Can you work these out from the model? Positions are in its coordinate system, mm. A direction names the side the tool comes from. Give positions to 0.01 mm unless a question says otherwise; leave off trailing zeros. Loops run counter-clockwise (first coordinate to the right, second up) from the corner with the lowest first, then second, coordinate; pieces in that order, holes last. Notation, with made-up numbers: (83, -33.5) - (104, -33.5) arc R32 cw to (104, -4.5) - close; hole circle Ø11 at (4, -9.5). An arc over 180 degrees is marked (long way). Write item = value, one per line.
Autodesk Inventor part; units mm, degrees
ref_plane "YZ Plane" through (0, 0, 0) normal (1, 0, 0) x (0, 1, 0)
ref_plane "XZ Plane" through (0, 0, 0) normal (0, 1, 0) x (-1, 0, 0)
ref_plane "XY Plane" through (0, 0, 0) normal (0, 0, 1) x (1, 0, 0)
sketch "Sketch1" plane through (0, 0, 0) normal (1, 0, 0) x (0, 1, 0)
  line L0 (-1.5, 6.858) -> (1.5, 6.858)
  line L1 (1.5, 6.858) -> (1.5, -6.858)
  line L2 (1.5, -6.858) -> (-1.5, -6.858)
  line L3 (-1.5, -6.858) -> (-1.5, 6.858)
  line L4 (-1.5, 6.858) -> (1.5, -6.858) construction
  line L5 (1.5, 6.858) -> (-1.5, -6.858) construction
  line L6 (1.5, 6.858) -> (39.5, 6.858)
  line L7 (39.5, 6.858) -> (39.5, 9.858)
  line L8 (39.5, 9.858) -> (1.5, 9.858)
  line L9 (1.5, 9.858) -> (1.5, 6.858)
  line L10 (1.5, -6.858) -> (39.5, -6.858)
  line L11 (39.5, -6.858) -> (39.5, -9.858)
  line L12 (39.5, -9.858) -> (1.5, -9.858)
  line L13 (1.5, -9.858) -> (1.5, -6.858)
  line L14 (9.5, 6.858) -> (1.5, 6.858)
  line L15 (1.5, 6.858) -> (1.5, -0.142)
  line L16 (1.5, -0.142) -> (9.5, -0.142)
  line L17 (9.5, -0.142) -> (9.5, 6.858)
  line L18 (9.5, -6.858) -> (1.5, -6.858)
  line L19 (1.5, -6.858) -> (1.5, -0.142)
  line L20 (1.5, -0.142) -> (9.5, -0.142)
  line L21 (9.5, -0.142) -> (9.5, -6.858)
  line L22 (9.5, -0.142) -> (1.5, -0.142)
  line L23 (1.5, 6.858) -> (-1.5, 6.858)
  line L24 (-1.5, 6.858) -> (-1.5, 9.858)
  line L25 (-1.5, 9.858) -> (1.5, 9.858)
  line L26 (1.5, 9.858) -> (1.5, 6.858)
  line L27 (1.5, -6.858) -> (-1.5, -6.858)
  line L28 (-1.5, -6.858) -> (-1.5, -9.858)
  line L29 (-1.5, -9.858) -> (1.5, -9.858)
  line L30 (1.5, -9.858) -> (1.5, -6.858)
  point P0 (0, 0)
  dimension "d0" = 3
  dimension "d2" = 13.716
  dimension "d3" = 3
  dimension "d4" = 3
  dimension "d5" = 38
  dimension "d6" = 38
  dimension "d7" = 0
  dimension "d8" = 8
  dimension "d9" = 8
  dimension "d12" = 7
  dimension "d13" = 6.716
extrude "Extrusion1" add sketch "Sketch1" along normal blind 45
sketch "Sketch2" plane through (0, -1.5, 9.858) normal (0, 0, 1) x (1, 0, 0)
  line L0 (5, 7) -> (8.9446, 7)
  arc A0 (5, 7) -> (5, 0) centre (5, 3.5) ccw
  line L1 (8.9446, 0) -> (5, 0)
  arc A1 (13.3822, 14.1239) -> (31.6178, 14.1239) centre (22.5, 3.5) ccw
  line L2 (13.3822, 14.1239) -> (13.3822, 15.7096)
  line L3 (13.6751, 16.4167) -> (15.15, 17.8916)
  arc A2 (13.6751, 16.4167) -> (13.3822, 15.7096) centre (14.3822, 15.7096) ccw
  arc A3 (16.15, 20.3916) -> (15.15, 19.3916) centre (16.15, 19.3916) ccw
  line L4 (15.15, 19.3916) -> (15.15, 17.8916)
  line L5 (28.85, 20.3916) -> (16.15, 20.3916)
  arc A4 (29.85, 19.3916) -> (28.85, 20.3916) centre (28.85, 19.3916) ccw
  line L6 (29.85, 17.8916) -> (29.85, 19.3916)
  line L7 (31.3249, 16.4167) -> (29.85, 17.8916)
  line L8 (31.6178, 15.7096) -> (31.6178, 14.1239)
  arc A5 (31.6178, 15.7096) -> (31.3249, 16.4167) centre (30.6178, 15.7096) ccw
  line L9 (40, 7) -> (36.0554, 7)
  arc A6 (40, 0) -> (40, 7) centre (40, 3.5) ccw
  line L10 (36.0554, 0) -> (40, 0)
  line L11 (40, 7) -> (36.0554, 7)
  arc A7 (40, 0) -> (40, 7) centre (40, 3.5) ccw
  line L12 (36.0554, 0) -> (40, 0)
  line L13 (8.9446, 0) -> (5, 0)
  line L14 (36.0554, 0) -> (40, 0)
  line L15 (0, 41) -> (0, 0)
  line L16 (0, 0) -> (45, 0)
  line L17 (45, 41) -> (45, 0)
  line L18 (0, 41) -> (45, 41)
  line L19 (5, 7) -> (8.9446, 7)
  arc A8 (5, 7) -> (5, 0) centre (5, 3.5) ccw
sketch "Sketch3" plane through (0, -1.5, 9.858) normal (0, 0, 1) x (1, 0, 0)
  line L0 (0, 0) -> (45, 0)
  line L1 (45, 41) -> (45, 0)
  point P0 (0, 41)
  point P1 (0, 1.5)
  point P2 (5, 3.5)
  point P3 (40, 3.5)
  dimension "d16" = 35
  dimension "d18" = 5
  dimension "d19" = 45
  dimension "d20" = 3.5
  dimension "d21" = 3.5
hole "Hole1" at (5, 2, 9.858) at (40, 2, 9.858) direction (0, 0, -1) diameter 4.2 end through all
extrude "Extrusion2" cut sketch "Sketch2" against normal blind 0.82 contours A1 L2 A2 L3 L4 A3 L5 A4 L6 L7 A5 L8 L16 | L16 A1
sketch "Sketch4" plane through (0, -1.5, 9.858) normal (0, 0, 1) x (1, 0, 0)
  arc A0 (36.0554, 0) -> (31.6178, 14.1239) centre (22.5, 3.5) ccw
  line L0 (36.0554, 0) -> (45, 0)
  arc A1 (13.3822, 14.1239) -> (8.9446, 0) centre (22.5, 3.5) ccw
  circle A2 centre (5, 3.5) radius 2.1
  circle A3 centre (40, 3.5) radius 2.1
  arc A4 (5, 7) -> (5, 0) centre (5, 3.5) ccw
  line L1 (5, 7) -> (8.9446, 7)
  line L2 (8.9446, 0) -> (5, 0)
  arc A5 (13.3822, 14.1239) -> (31.6178, 14.1239) centre (22.5, 3.5) ccw
  arc A6 (13.3822, 14.1239) -> (31.6178, 14.1239) centre (22.5, 3.5) ccw
  line L3 (40, 7) -> (36.0554, 7)
  arc A7 (40, 0) -> (40, 7) centre (40, 3.5) ccw
  line L4 (36.0554, 0) -> (40, 0)
  point P0 (0, 1.5)
extrude "Extrusion3" cut sketch "Sketch4" against normal blind 0.82
sketch "Sketch5" plane through (0, -1.5, -9.858) normal (0, 0, -1) x (-1, 0, 0)
  circle A0 centre (-5, 3.5) radius 2.1
  circle A1 centre (-40, 3.5) radius 2.1
  line L0 (-34.959, 3.5) -> (-37.4795, -0.8656)
  line L1 (-37.4795, -0.8656) -> (-42.5205, -0.8656)
  line L2 (-42.5205, -0.8656) -> (-45.041, 3.5)
  line L3 (-45.041, 3.5) -> (-42.5205, 7.8656)
  line L4 (-42.5205, 7.8656) -> (-37.4795, 7.8656)
  line L5 (-37.4795, 7.8656) -> (-34.959, 3.5)
  line L6 (0.041, 3.5) -> (-2.4795, -0.8656)
  line L7 (-2.4795, -0.8656) -> (-7.5205, -0.8656)
  line L8 (-7.5205, -0.8656) -> (-10.041, 3.5)
  line L9 (-10.041, 3.5) -> (-7.5205, 7.8656)
  line L10 (-7.5205, 7.8656) -> (-2.4795, 7.8656)
  line L11 (-2.4795, 7.8656) -> (0.041, 3.5)
  point P0 (0, 1.5)
  point P1 (-40, 3.5)
  point P2 (-5, 3.5)
  dimension "d33" = 8.7312
  dimension "d34" = 8.7312
extrude "Extrusion4" cut sketch "Sketch5" against normal blind 3.175
sketch "Sketch6" plane through (0, 9.5, 6.858) normal (0, 1, 0) x (1, 0, 0)
  line L0 (7.5, 1.82) -> (37.5, 1.82)
  line L1 (37.5, 9.82) -> (7.5, 9.82)
  line L2 (7.5, 1.82) -> (7.5, 9.82)
  line L3 (37.5, 1.82) -> (37.5, 9.82)
  line L4 (7, 10.32) -> (38, 10.32)
  line L5 (38, 10.32) -> (38, 1.32)
  line L6 (38, 1.32) -> (7, 1.32)
  line L7 (7, 1.32) -> (7, 10.32)
  line L8 (8, 10.32) -> (37, 10.32)
  line L9 (37, 10.32) -> (37, 1.32)
  line L10 (37, 1.32) -> (8, 1.32)
  line L11 (8, 1.32) -> (8, 10.32)
  line L12 (0, 0) -> (45, 0)
  line L13 (8, 1.32) -> (37, 1.32)
  line L14 (37, 1.32) -> (37, 0)
  line L15 (37, 0) -> (8, 0)
  line L16 (8, 0) -> (8, 1.32)
  point P0 (0, 6.858)
  dimension "d37" = 0.5
  dimension "d56" = 1
  dimension "d57" = 1
chamfer "Chamfer1" distance 1 angle 45 2 edges at (22.5, 39.5, -6.858) (22.5, 39.5, 6.858)
sketch "Sketch7" plane through (0, 9.5, -6.858) normal (0, 0, 1) x (1, 0, 0)
  line L0 (0, 29) -> (0, 0)
  line L1 (0, 0) -> (45, 0)
  line L2 (45, 29) -> (45, 0)
  circle A0 centre (22.5, 10) radius 4.318
  line L3 (22.5, 10) -> (22.5, 20)
  circle A1 centre (22.5, 20) radius 2.159
  line L4 (20.341, 20) -> (20.341, 6.2605)
  line L5 (24.659, 20) -> (24.659, 6.2605)
  point P0 (0, -9.5)
  dimension "d43" = 8.636
  dimension "d45" = 10
  dimension "d46" = 4.318
  dimension "d47" = 22.5
  dimension "d48" = 45
  dimension "d49" = 10
extrude "Extrusion6" cut sketch "Sketch7" against normal through all
sketch "Sketch8" plane through (0, 9.5, -6.858) normal (0, 0, 1) x (1, 0, 0)
  arc A0 (20.341, 13.7395) -> (24.659, 13.7395) centre (22.5, 10) ccw
  line L0 (20.341, 13.7395) -> (20.341, 20)
  arc A1 (24.659, 20) -> (20.341, 20) centre (22.5, 20) ccw
  line L1 (24.659, 20) -> (24.659, 13.7395)
  line L2 (45, 29) -> (45, 0)
  circle A2 centre (22.5, 20) radius 4.318
  line L3 (18.182, 20) -> (18.182, 10)
  line L4 (26.818, 10) -> (26.818, 20)
  point P0 (0, -9.5)
  dimension "d52" = 4.318
  dimension "d53" = 8.636
extrude "Extrusion7" cut sketch "Sketch8" against normal blind 2 contours L0 A2 L1 A0 | A0 L3 A2 L0 | A2 L1 A1 L0 | A0 L1 A2 L4 picked at (24.9024, 17.6839)
extrude "Extrusion8" cut sketch "Sketch6" against normal through all contours L11 L1 L9 L0 | L0 L9 L6 L11 | L6 L14 L12 L16 | L11 L4 L9 L1
sketch "Sketch9" plane through (0, 0, 0) normal (-1, 0, 0) x (0, 0, 1)
  line L0 (37.1954, 50) -> (6.858, 50)
  line L1 (6.858, 50) -> (6.858, -18)
  line L2 (6.858, -18) -> (37.1954, -18)
  line L3 (37.1954, -18) -> (37.1954, 50)
  point P0 (0, 0)
extrude "Extrusion9" cut sketch "Sketch9" against normal through all
sketch "Sketch10" plane through (0, -1.5, 6.858) normal (0, 0, 1) x (1, 0, 0)
  line L0 (0, 11) -> (8, 11)
  line L1 (0, 0) -> (0, 11)
  line L2 (8, 0) -> (0, 0)
  line L3 (8, 11) -> (8, 0)
  circle A0 centre (5, 3.5) radius 2.1
  line L4 (7.5, 10.5) -> (0.5, 10.5)
  line L5 (0.5, 10.5) -> (0.5, 0.5)
  line L6 (0.5, 0.5) -> (7.5, 0.5)
  line L7 (7.5, 0.5) -> (7.5, 10.5)
  point P0 (0, 1.5)
  dimension "d62" = 0.5
extrude "Extrusion10" add sketch "Sketch10" along normal blind 3 contours L0 L3 L2 L1 | L7 L6 L5 L4
sketch "Sketch11" plane through (37, -1.5, 6.858) normal (0, 0, 1) x (1, 0, 0)
  line L0 (0, 11) -> (0, 0)
  line L1 (8, 0) -> (0, 0)
  line L2 (8, 11) -> (8, 0)
  line L3 (0, 11) -> (8, 11)
  circle A0 centre (3, 3.5) radius 2.1
  line L4 (7.5, 10.5) -> (7.5, 0.5)
  line L5 (7.5, 0.5) -> (0.5, 0.5)
  line L6 (0.5, 0.5) -> (0.5, 10.5)
  line L7 (0.5, 10.5) -> (7.5, 10.5)
  point P0 (-37, 1.5)
  dimension "d65" = 0.5
extrude "Extrusion11" add sketch "Sketch11" along normal blind 3 contours L3 L2 L1 L0 | L4 L5 L6 L7
sketch "Sketch12" plane through (0, -1.5, 9.858) normal (0, 0, 1) x (1, 0, 0)
  circle A0 centre (5, 3.5) radius 2.1
  circle A1 centre (40, 3.5) radius 2.1
  circle A2 centre (5, 3.5) radius 2.1
  line L0 (40, 0) -> (5, 0)
  arc A3 (40, 0) -> (40, 7) centre (40, 3.5) ccw
  line L1 (36.0554, 7) -> (40, 7)
  arc A4 (36.0554, 7) -> (31.6178, 14.1239) centre (22.5, 3.5) ccw
  line L2 (31.6178, 15.7096) -> (31.6178, 14.1239)
  arc A5 (31.6178, 15.7096) -> (31.3249, 16.4167) centre (30.6178, 15.7096) ccw
  line L3 (29.85, 17.8916) -> (31.3249, 16.4167)
  line L4 (29.85, 19.3916) -> (29.85, 17.8916)
  arc A6 (29.85, 19.3916) -> (28.85, 20.3916) centre (28.85, 19.3916) ccw
  line L5 (16.15, 20.3916) -> (28.85, 20.3916)
  arc A7 (16.15, 20.3916) -> (15.15, 19.3916) centre (16.15, 19.3916) ccw
  line L6 (15.15, 17.8916) -> (15.15, 19.3916)
  line L7 (13.6751, 16.4167) -> (15.15, 17.8916)
  arc A8 (13.6751, 16.4167) -> (13.3822, 15.7096) centre (14.3822, 15.7096) ccw
  line L8 (13.3822, 14.1239) -> (13.3822, 15.7096)
  arc A9 (13.3822, 14.1239) -> (8.9446, 7) centre (22.5, 3.5) ccw
  line L9 (5, 7) -> (8.9446, 7)
  arc A10 (5, 7) -> (5, 0) centre (5, 3.5) ccw
  point P0 (0, 1.5)
extrude "Extrusion12" cut sketch "Sketch12" against normal blind 0.82
sketch "Sketch13" plane through (0, 9.5, -6.858) normal (0, 1, 0) x (1, 0, 0)
  line L0 (37, -3.396) -> (37, -16.716)
  line L1 (8, -16.716) -> (8, -3.396)
  line L2 (45, -14.716) -> (45, -13.716)
  line L3 (45, -13.716) -> (0, -13.716)
  line L4 (0, -13.716) -> (0, -14.716)
  line L5 (0, -14.716) -> (45, -14.716)
  line L6 (8, -10.056) -> (10.1131, -13.716)
  line L7 (37, -10.056) -> (34.8869, -13.716)
  line L8 (37, -10.056) -> (37, -13.716)
  line L9 (37, -13.716) -> (34.8869, -13.716)
  line L10 (10.1131, -13.716) -> (8, -13.716)
  line L11 (8, -13.716) -> (8, -10.056)
  point P0 (0, -6.858)
  dimension "d70" = 30
  dimension "d71" = 30
extrude "Extrusion13" add sketch "Sketch13" against normal blind 8 contours L0 L3 L7 | L3 L1 L6
equation "\"d2\" = StretcherDepth"
equation "\"d6\" = d5"
equation "\"d9\" = d8"
equation "\"d47\" = 0.5 * d48"
equation "\"d53\" = 2 * d52"
properties part number "MotorClipV3Back" material "ABS Plastic"
Q1. Imagine slicing it at A-A, the plane z = -1. Write out the boundary of the cut face in (x, y).
Output:
outline = (0, -1.5) - (8, -1.5) - (8, 9.5) - (0, 9.5) - close; (37, -1.5) - (45, -1.5) - (45, 9.5) - (37, 9.5) - close; hole circle Ø4.2 at (5, 2); hole circle Ø4.2 at (40, 2)
Q2. Imagine slicing it at D-D, the plane z = -5. Write out the boundary of the cut face in (x, y).
Output:
outline = (0, -1.5) - (45, -1.5) - (45, 9.5) - (0, 9.5) - close; hole circle Ø4.2 at (5, 2); hole circle Ø4.2 at (40, 2)
Q3. I need wall thicknesses on L1, parallel to X at y = 2, z = 0.5; L2, parallel to Y at x = 40, z = 6.25; L3, parallel to X at y = 19.5, z = -9.5. Which ranges of each line are inside material? Lowest first, please.
Output:
L1 = 0 to 2.9, 7.1 to 8, 37 to 37.9, 42.1 to 45
L2 = -1.5 to -0.1, 4.1 to 9.5
L3 = 0 to 18.18, 26.82 to 45
Q4. We'd pull the mould along Y, two halves only. Please class faces 4 (the flat face through (37, 4, 3)), 5 (the cylindrical face through (43.5, 1.9, 9.5)), 6 (the flat face through (22, 9.5, -4)), 7 (the flat face through (36, 1.5, 6)): released by +Y, released by -Y, zero draft, split by the parting line, or undercut.
Output:
face_4 = zero draft
face_5 = undercut
face_6 = released by +Y
face_7 = released by -Y
Q5. Imagine slicing it at C-C, the plane x = 22.5. Write out the boundary of the cut face in (y, z), then the cut area to 3 significant figures.
Output:
outline = (-1.5, -9.86) - (15.18, -9.86) - (15.18, -6.86) - (9.5, -6.86) - (9.5, -3.46) - (-1.5, -3.46) - close; (31.66, -9.86) - (39.5, -9.86) - (39.5, -7.86) - (38.5, -6.86) - (33.82, -6.86) - (33.82, -8.86) - (31.66, -8.86) - close
area = 106 mm2
Q6. Which directions (+Z, -Z, +X, -X, +Y, -Y) give clear straight access to the entire face, cutting with the end or side of a thin tool? Please do faces 1 (the flat face through (5, 6.366, -8)), 2 (the flat face through (18.182, 25, -8)), 3 (the flat face through (38.9, 4.2, -6.683)).
Output:
face_1 = -Z, -Y
face_2 = +Z
face_3 = -Z
Q7. For pin 1 (5.5 mm diameter, centred on x = 27, y = 6.5, fed in from +Z); pin 2 (1.7 mm diameter, centred on x = 9.5, z = 5, fed in from -Y); pin 3 (6 mm diameter, centred on x = 8, z = 6, fed in from +Y); pin 4 (3 mm diameter, centred on x = 5, y = 1.5, fed in from +Z), each with a flat end and sliding along its axis, tell me the tip position at first contact or that it passes through.
Output:
pin_1 = -3.46
pin_2 = 1.5
pin_3 = 9.5
pin_4 = through
Q8. Imagine slicing it at B-B, the plane y = 25. Write out the boundary of the cut face in (x, z), then the cut area to 3 significant figures.
Output:
outline = (0, -9.86) - (20.34, -9.86) - (20.34, -8.86) - (18.18, -8.86) - (18.18, -6.86) - (0, -6.86) - close; (24.66, -9.86) - (45, -9.86) - (45, -6.86) - (26.82, -6.86) - (26.82, -8.86) - (24.66, -8.86) - close
area = 113 mm2
